```python
from build123d import *

# Parameters (mm, degrees)
SKETCH_R      = 35
PAD_DEPTH     = 30
SKETCH001_R   = 33.5
POCKET_DEPTH  = 30.001
SKETCH002_R   = 80
SKETCH002_R_2 = 35
PAD001_DEPTH  = 4


with BuildPart() as part:
    # Sketch → Pad (new body)
    with BuildSketch(Plane.XY):
        Circle(SKETCH_R)
    extrude(amount=PAD_DEPTH)

    # Sketch001 → Pocket (cut, through all)
    with BuildSketch(Plane.XY):
        Circle(SKETCH001_R)
    extrude(amount=POCKET_DEPTH, mode=Mode.SUBTRACT)

    # Sketch002 (on DatumPlane) → Pad001 (join)
    with BuildSketch(Plane.XY.offset(30)):
        Circle(SKETCH002_R)
        Circle(SKETCH002_R_2, mode=Mode.SUBTRACT)
    extrude(amount=-PAD001_DEPTH)


solid = part.part
```
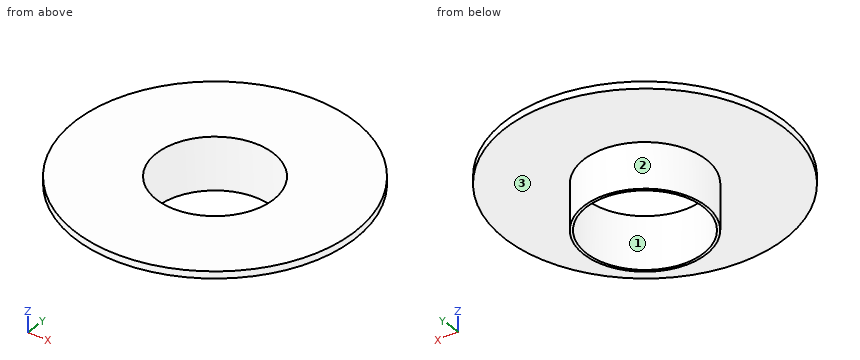
Input: part model. Units: mm. Frame: model coordinates. Face numbers are marked on the shaded views. Give positions to 0.01 mm unless a question says otherwise; leave off trailing zeros. Write each loop counter-clockwise with the first axis right and the second up, starting at its lowest first coordinate (ties: lowest second). Pieces come first, ordered by that corner, then holes. Notation, with made-up numbers: (14.5, 30) - (67.5, 30) arc R35 cw to (67.5, 67) - close; hole circle Ø3 at (78.5, -36). An arc over 180 degrees is marked (long way). Write item = value, one per line. Start each with the question number.
1) Cut plane C-C (z = 15.5). Return loops of the section in (x, y), and give its area (3 significant figures).
2) Draft query along Y for the marked faces 1, 2 and 3. Return one class per face: pulls with the +Y half, pulls with the -Y half, needs draft (parallel to the pull), parting line crosses it, or undercut.
3) Material intervals for L1, parallel to Y at x = 0, z = 8; L2, parallel to Z at x = -28.5, y = -35.5; L3, parallel to X at y = 8, z = 24, sorted ascending. Write a range as [from, to].
4) Pin query (flat end, axial travel): pin 1 (12 mm diameter, centred on y = -31, z = 10.5, fed in from +X); pin 2 (2 mm diameter, centred on x = 32.5, z = 13, fed in from +Y); pin 3 (1 mm diameter, centred on y = -13.5, z = 3.5, fed in from +X). Return the tip coordinate at first contact, or that it passes through.
5) Cut plane D-D (y = 54). Return loops of the section in (x, z).
6) Cut plane A-A (x = 0). Return loops of the section in (y, z), and give its area (3 significant figures).
Answers follow:
q1.outline = circle Ø70 at (0, 0); hole circle Ø67 at (0, 0)
q1.area = 323 mm^2
q2.face_1 = undercut
q2.face_2 = parting line crosses it
q2.face_3 = needs draft
q3.L1 = [-35, -33.5], [33.5, 35]
q3.L2 = [26, 30]
q3.L3 = [-34.07, -32.53], [32.53, 34.07]
q4.pin_1 = 24.49
q4.pin_2 = 15.26
q4.pin_3 = 32.5
q5.outline = (-59.03, 26) - (59.03, 26) - (59.03, 30) - (-59.03, 30) - close
q6.outline = (-80, 26) - (-35, 26) - (-35, 0) - (-33.5, 0) - (-33.5, 30) - (-80, 30) - close; (33.5, 0) - (35, 0) - (35, 26) - (80, 26) - (80, 30) - (33.5, 30) - close
q6.area = 450 mm^2
